Work out the finished part from the listing and answer in its coordinate system (mm). A direction names the side the tool comes from. Give positions to 0.01 mm unless a question says otherwise; leave off trailing zeros. Write each loop counter-clockwise with the first axis right and the second up, starting at its lowest first coordinate (ties: lowest second). Pieces come first, ordered by that corner, then holes.
1) Straight lines are drawn through the part: probe 1 along Y at (x, z) = (148.5, 69.5); probe 2 along X at (y, z) = (69.5, 141); probe 3 along Y at (x, z) = (43.5, 10.5). For each, find the intervals that lie inside material, in ascending order.
2) Determine the mould class of faces 4 (the face through (129, 37.5, 81)), 5 (the face through (132, 2, 1)), 6 (the face through (128, 113, 159)) for opening direction Y: pulls with the +Y half, pulls with the -Y half, needs draft (parallel to the pull), parting line crosses it, or undercut.
3) Find section A-A (z = 141.5). Determine the outline of the cut face in (x, y).
4) A tool of negligible diameter and unlimited length cuts with its end or side. For faces 1 (the face through (131.12, 79, 158.57)), 2 (the face through (229.995, 57.06, 81.05)), 3 (the face through (128.88, 79, 1.43)), from which of +Z, -Z, +X, -X, +Y, -Y can it reach the whole face along a straight path? Write none if from no direction.
5) Find section C-C (x = 64). Determine the outline of the cut face in (y, z).
6) Find section B-B (y = 57.5). Determine the outline of the cut face in (x, z).
```python
from build123d import *

# Parameters (mm, degrees)
SKETCH_W     = 260
SKETCH_H     = 115
PAD_DEPTH    = 160
POCKET_DEPTH = 160.001
FILLET_R     = 10
FILLET001_R  = 5


with BuildPart() as part:
    # Sketch → Pad (new body)
    with BuildSketch(Plane.XY):
        with Locations((130, 57.5)):
            Rectangle(SKETCH_W, SKETCH_H)
    extrude(amount=PAD_DEPTH)

    # Sketch001 → Pocket (cut, through all)
    with BuildSketch(Plane.XY.offset(160)):
        with BuildLine():
            ThreePointArc((50, 77.5), (30, 57.5), (50, 37.5))
            Line((50, 37.5), (210, 37.5))
            ThreePointArc((210, 37.5), (230, 57.5), (210, 77.5))
            Line((50, 77.5), (210, 77.5))
        make_face()
    extrude(amount=-POCKET_DEPTH, mode=Mode.SUBTRACT)

    # Fillet
    fillet_edges = [part.edges().sort_by_distance(p)[0] for p in [
        (0, 0, 80),
        (0, 115, 80),
        (260, 0, 80),
        (260, 115, 80),
    ]]
    fillet(fillet_edges, radius=FILLET_R)

    # Fillet001
    fillet001_edges = [part.edges().sort_by_distance(p)[0] for p in [
        (130, 0, 0),
        (2.928932, 2.928932, 0),
        (257.071068, 2.928932, 0),
        (0, 57.5, 0),
        (260, 57.5, 0),
        (2.928932, 112.071068, 0),
        (257.071068, 112.071068, 0),
        (130, 115, 0),
        (130, 37.5, 0),
        (30, 57.5, 0),
        (130, 77.5, 0),
        (230, 57.5, 0),
        (130, 0, 160),
        (2.928932, 2.928932, 160),
        (257.071068, 2.928932, 160),
        (0, 57.5, 160),
        (260, 57.5, 160),
        (2.928932, 112.071068, 160),
        (257.071068, 112.071068, 160),
        (130, 115, 160),
        (130, 77.5, 160),
        (230, 57.5, 160),
        (130, 37.5, 160),
        (30, 57.5, 160),
    ]]
    fillet(fillet001_edges, radius=FILLET001_R)


solid = part.part
```
Results:
1. probe 1: y = 0 to 37.5, 77.5 to 115
1. probe 2: x = 0 to 34, 226 to 260
1. probe 3: y = 0 to 38.59, 76.41 to 115
2. face 4: undercut
2. face 5: pulls with the -Y half
2. face 6: pulls with the +Y half
3. outline: (0, 10) arc R10 ccw to (10, 0) - (250, 0) arc R10 ccw to (260, 10) - (260, 105) arc R10 ccw to (250, 115) - (10, 115) arc R10 ccw to (0, 105) - close; hole (50, 37.5) - (210, 37.5) arc R20 ccw to (210, 77.5) - (50, 77.5) arc R20 ccw to start
4. face 1: +Z
4. face 2: +Z, -Z
4. face 3: -Z
5. outline: (0, 5) arc R5 ccw to (5, 0) - (32.5, 0) arc R5 ccw to (37.5, 5) - (37.5, 155) arc R5 ccw to (32.5, 160) - (5, 160) arc R5 ccw to (0, 155) - close; (77.5, 5) arc R5 ccw to (82.5, 0) - (110, 0) arc R5 ccw to (115, 5) - (115, 155) arc R5 ccw to (110, 160) - (82.5, 160) arc R5 ccw to (77.5, 155) - close
6. outline: (0, 5) arc R5 ccw to (5, 0) - (25, 0) arc R5 ccw to (30, 5) - (30, 155) arc R5 ccw to (25, 160) - (5, 160) arc R5 ccw to (0, 155) - close; (230, 5) arc R5 ccw to (235, 0) - (255, 0) arc R5 ccw to (260, 5) - (260, 155) arc R5 ccw to (255, 160) - (235, 160) arc R5 ccw to (230, 155) - close
